Read the model definition and answer for the solid it produces. Units are mm, in the model's axes. Give positions to 0.01 mm unless a question says otherwise; leave off trailing zeros.
(1) Determine the mould class of faces 1 (the face through (-65.4, 53.98, -104.57)), 2 (the face through (-64.772, 51.456, -159.795)), 3 (the face through (-65, 66.675, -128)) for opening direction Y: pulls with the +Y half, pulls with the -Y half, needs draft (parallel to the pull), parting line crosses it, or undercut.
(2) Straight lines are drawn through the part: probe 1 along Y at (x, z) = (-61, -104.5); probe 2 along Z at (x, y) = (-81.5, 57.5) (3 decimals); probe 3 along Z at (x, y) = (-49, 59) (3 decimals). For each, find the intervals that lie inside material, in ascending order.
(3) Find section A-A, the plane x = -82. State how many separate pieces and enclosed holes the cut face has, then the cut area to 3 significant figures.
(4) Each of these flat-tipped pins is pushed along its axis until it touches: P1, Ø4, axis at x = -76.5, y = 62.5, coming from the +Z side; P2, Ø7.5, axis at y = 58.74, z = -144.15, coming from the -X side; P3, Ø6, axis at x = -79.5, z = -93.5, coming from the +Y side; P4, Ø5, axis at x = -52.5, y = 56, coming from the -Z side. Where does it stop, or does it pass through?
```python
from build123d import *

# Parameters (mm, degrees)
STOCK_HAMMERSAW_START                 = -88.9
STOCK_HAMMERSAW_MULTIBODY_1_OUTLINE_R = 4.7625
STOCK_HAMMERSAW_MULTIBODY_1_DEPTH     = 47.625
FILLET1_R                             = 1.27
CHAMFER1_SIZE                         = 1.27


# Read off the part's stored shape, not the designer's step: Stock-HammerSaw Multibody-1
with BuildPart() as part:
    # Stock-HammerSaw Multibody-1 outline → Stock-HammerSaw Multibody-1 (new body)
    with BuildSketch(Plane.YZ.offset(STOCK_HAMMERSAW_START)):
        with BuildLine():
            Line((66.675, -151.571456433), (66.675, -104.775))
            ThreePointArc((66.675, -104.775), (65.121562553, -85.476521096), (60.501252996, -66.675))
            Line((60.501252996, -66.675), (50.8, -66.675))
            Line((50.8, -66.675), (50.8, -160.903282658))
            Line((50.8, -160.903282658), (66.675, -151.571456433))
        make_face()
        with Locations((58.7375, -144.145)):
            Circle(STOCK_HAMMERSAW_MULTIBODY_1_OUTLINE_R, mode=Mode.SUBTRACT)
        with Locations((58.7375, -104.775)):
            Circle(STOCK_HAMMERSAW_MULTIBODY_1_OUTLINE_R, mode=Mode.SUBTRACT)
    extrude(amount=STOCK_HAMMERSAW_MULTIBODY_1_DEPTH)

    # Fillet1
    fillet1_edges = [part.edges().sort_by_distance(p)[0] for p in [
        (-65.0875, 66.675, -151.571456433),
        (-65.0875, 50.8, -160.903282658),
        (-65.0875, 50.8, -66.675),
        (-65.0875, 60.501252996, -66.675),
    ]]
    fillet(fillet1_edges, radius=FILLET1_R)

    # Chamfer1
    chamfer1_edges = [part.edges().sort_by_distance(p)[0] for p in [
        (-41.275, 53.975, -144.145),
        (-41.275, 53.975, -104.775),
        (-88.9, 65.194617982, -85.932902187),
        (-88.9, 53.975, -144.145),
        (-88.9, 53.975, -104.775),
        (-88.9, 50.8, -113.314283072),
        (-41.275, 50.8, -113.314283072),
        (-41.275, 55.825875065, -66.675),
        (-41.275, 59.381087146, -155.859048701),
        (-41.275, 66.675, -127.809916057),
        (-41.275, 51.171974388, -67.046974388),
        (-41.275, 60.328510865, -66.917747157),
        (-41.275, 66.507328371, -151.475523927),
        (-41.275, 51.439308188, -159.785894515),
        (-88.9, 59.381087146, -155.859048701),
        (-88.9, 66.675, -127.809916057),
        (-88.9, 55.825875065, -66.675),
        (-88.9, 51.171974388, -67.046974388),
        (-88.9, 60.328510865, -66.917747157),
        (-88.9, 66.507328371, -151.475523927),
        (-88.9, 51.439308188, -159.785894515),
        (-41.275, 65.194617982, -85.932902187),
    ]]
    chamfer(chamfer1_edges, length=CHAMFER1_SIZE)


solid = part.part
```
Entries:
1. face 1: undercut
1. face 2: parting line crosses it
1. face 3: pulls with the +Y half
2. probe 1: y = 50.8 to 53.98, 63.49 to 66.67
2. probe 2: z = -156.965 to -148.744, -139.546 to -109.374, -100.176 to -66.675
2. probe 3: z = -156.083 to -148.9, -139.39 to -109.53, -100.02 to -66.675
3. separate pieces: 1
3. enclosed holes: 2
3. area: 1,200 mm2
4. P1: stops at z = -67.07
4. P2: passes through
4. P3: stops at y = 66.39
4. P4: stops at z = -159.32
